Model file for the job. Use its own axes, mm. Face numbers are marked on the shaded views. A direction names the side the tool comes from. Round coordinates to 2 decimals unless told otherwise and drop trailing zeros. Loops run counter-clockwise (first coordinate to the right, second up) from the corner with the lowest first, then second, coordinate; pieces in that order, holes last. Notation, with made-up numbers: M 12,-6 L 33,-6 A9 ccw 33,4 Z; hole C 33.25,48.5 d9. An arc over 180 degrees is marked long. Use a Markdown table: item, result. Add a question column.
Q1. Pin check, flat tips, straight feed: pin 1 (12 mm diameter, centred on x = -80, z = 150.5, fed in from +Y); pin 2 (6 mm diameter, centred on x = -57.5, z = 228, fed in from -Y); pin 3 (10 mm diameter, centred on x = -74.5, y = 64, fed in from +Z). Stop position of each tip, or through.
Q2. Tool access for the marked faces 1 and 2: list every direction of +Z, -Z, +X, -X, +Y, -Y with a clear straight run to the whole face (end or side of a thin tool).
Q3. Cut at B-B (z = 240). Give the cut face in (x, y), plus the area to 3 significant figures.
Q4. Probe line 1 (Y direction, x = -7, z = 102); line 2 (Z direction, x = -56.5, y = 75.5); line 3 (Z direction, x = -29, y = 55). List the from-to ranges inside material, lowest first. Write a range as from..to.
Q5. Cut at D-D (y = 50). Give the cut face in (x, z).
Q6. Cut at A-A (y = 133.5). Give the cut face in (x, z), plus the area to 3 significant figures.
Q7. Cut at C-C (x = -58.5). Give the cut face in (y, z).
Q8. Mould opens along Y. For the marked faces 3, 4 and 5 say: +Y half, -Y half, draft (parallel to the pull), parting line (faces both ways), or undercut.
from build123d import *

# Parameters (mm, degrees)
BOSS_EXTRUDE1_DEPTH     = 229
SKETCH2_R               = 44.45
CUT_EXTRUDE1_DEPTH      = 78
SKETCH3_R               = 28.575
CUT_EXTRUDE2_DEPTH      = 243.326226397
CUT_EXTRUDE3_DEPTH      = 13
BOSS_EXTRUDE2_DEPTH     = 33
CUT_EXTRUDE4_REACH      = 325.365
CUT_EXTRUDE4_END_RADIUS = 28.575
SKETCH7_W               = 19
SKETCH7_H               = 33


with BuildPart() as part:
    # Sketch1 → Boss-Extrude1 (new body)
    with BuildSketch(Plane.XY):
        with BuildLine():
            Line((0, 0), (-13, 0))
            Line((-13, 0), (-95, 47.342722074))
            Line((-95, 47.342722074), (-95, 82))
            ThreePointArc((-95, 82), (-66.188344588, 144.409935107), (0, 162.962954492))
            Line((0, 162.962954492), (0, 0))
        make_face()
    extrude(amount=BOSS_EXTRUDE1_DEPTH)

    # Sketch2 → Cut-Extrude1 (cut)
    with BuildSketch(Plane.XY.offset(229)):
        with Locations((0, 81.481477246)):
            Circle(SKETCH2_R)
    extrude(amount=-CUT_EXTRUDE1_DEPTH, mode=Mode.SUBTRACT)

    # Sketch3 → Cut-Extrude2 (cut, through all)
    with BuildSketch(Plane.XY.offset(151)):
        with Locations((0, 81.481477246)):
            Circle(SKETCH3_R)
    extrude(amount=-CUT_EXTRUDE2_DEPTH, mode=Mode.SUBTRACT)

    # Sketch4 → Cut-Extrude3 (cut)
    with BuildSketch(Plane(origin=(0, 0, 0), x_dir=(0, 0, -1), z_dir=(1, 0, 0))):
        with BuildLine():
            Line((0, 15.453238623), (-114, 15.453238623))
            ThreePointArc((-114, 15.453238623), (-125, 26.453238623), (-114, 37.453238623))
            Line((-114, 37.453238623), (0, 37.453238623))
            ThreePointArc((0, 37.453238623), (11, 26.453238623), (0, 15.453238623))
        make_face()
    extrude(amount=-CUT_EXTRUDE3_DEPTH, mode=Mode.SUBTRACT)

    # Sketch5 → Boss-Extrude2 (add)
    with BuildSketch(Plane.XY.offset(229)):
        with BuildLine():
            Line((-37.972309742, 160.104953404), (-16.437525278, 143.280135832))
            Line((-16.437525278, 143.280135832), (-65.108558458, 80.984054183))
            Line((-65.108558458, 80.984054183), (-92.438236004, 102.336338426))
            ThreePointArc((-92.438236004, 102.336338426), (-72.663168997, 138.25216676), (-37.972309742, 160.104953404))
        make_face()
    extrude(amount=BOSS_EXTRUDE2_DEPTH)

    # Cut-Extrude4: up to this cylinder (the profile starts outside it)
    cut_extrude4_end = Plane(origin=(0, 81.481477246, 54.5), z_dir=(0, 0, 1)) * Cylinder(CUT_EXTRUDE4_END_RADIUS, 708.88, mode=Mode.PRIVATE)
    # Sketch7 → Cut-Extrude4 (cut, up to the surface)
    with BuildSketch(Plane(origin=(0, 164, 0), x_dir=(1, 0, 0), z_dir=(0, 1, 0)), mode=Mode.PRIVATE) as cut_extrude4_sk1:
        with Locations((-9.5, -54.5)):
            Rectangle(SKETCH7_W, SKETCH7_H)
    cut_extrude4_tool1 = extrude(cut_extrude4_sk1.sketch, amount=-CUT_EXTRUDE4_REACH, mode=Mode.PRIVATE) - cut_extrude4_end
    add(cut_extrude4_tool1.solids().sort_by_distance((-9.5, 164, 54.5))[0], mode=Mode.SUBTRACT)


solid = part.part
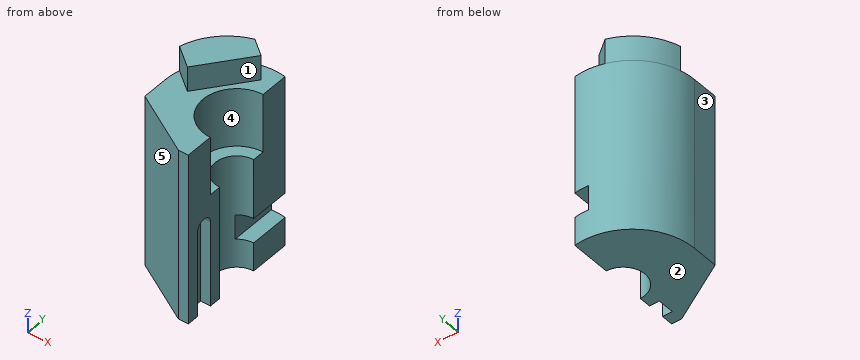
Checked values:
| question | item | result |
|---|---|---|
| 1 | pin 1 | stops at y = 136.8 |
| 1 | pin 2 | stops at y = 23.96 |
| 1 | pin 3 | stops at z = 229 |
| 2 | face 1 | +Z, +X, -Y |
| 2 | face 2 | -Z, +X, -X, +Y, -Y |
| 3 | outline | M -92.44,102.34 L -65.11,80.98 L -16.44,143.28 L -37.97,160.1 A82 ccw Z |
| 3 | area | 3,000 mm^2 |
| 4 | line 1 | y = 0..15.45, 37.45..53.78, 109.19..163.78 |
| 4 | line 2 | z = 0..229 |
| 4 | line 3 | z = 0..151 |
| 5 | outline | M -95,0 L 0,0 L 0,151 L -31.38,151 L -31.38,229 L -95,229 Z |
| 6 | outline | M -76.81,0 L 0,0 L 0,38 L -19,38 L -19,71 L 0,71 L 0,229 L -24.08,229 L -24.08,262 L -76.81,262 Z |
| 6 | area | 18,700 mm^2 |
| 7 | outline | M 26.27,0 L 150.22,0 L 150.22,262 L 89.44,262 L 89.44,229 L 26.27,229 Z |
| 8 | face 3 | draft |
| 8 | face 4 | undercut |
| 8 | face 5 | -Y half |
